Check sheet for the modelled part. Datum: model origin and axes. Units: mm. A direction names the side the tool comes from. Round coordinates to 2 decimals unless told otherwise and drop trailing zeros. Order: outer loops, then holes, each group sorted by start corner. A loop starts at its lowest first (then second) coordinate and runs counter-clockwise, first axis right, second up.
Autodesk Inventor part; units mm, degrees
ref_plane "YZ Plane" through (0, 0, 0) normal (1, 0, 0) x (0, 1, 0)
ref_plane "XZ Plane" through (0, 0, 0) normal (0, 1, 0) x (-1, 0, 0)
ref_plane "XY Plane" through (0, 0, 0) normal (0, 0, 1) x (1, 0, 0)
sketch "Skizze1" plane through (0, 0, 0) normal (0, 1, 0) x (-1, 0, 0)
  line L0 (39.8687, 22.5) -> (39.8687, 24)
  line L1 (39.8687, 24) -> (37.8687, 24)
  line L2 (37.8687, 24) -> (37.8687, 25)
  line L3 (37.8687, 25) -> (36.3687, 25)
  line L4 (36.3687, 22) -> (24.8687, 18.0718)
  line L5 (24.8687, 18.0718) -> (24.8687, 17.0718)
  line L6 (24.8687, 17.0718) -> (23.8687, 17.0718)
  line L7 (23.8687, 17.0718) -> (23.8687, 19)
  line L8 (23.8687, 19) -> (16.8687, 19)
  line L9 (16.8687, 19) -> (16.8687, 18)
  line L10 (16.8687, 18) -> (15.8687, 18)
  line L11 (15.8687, 18) -> (15.8687, 0)
  line L12 (39.8687, 22.5) -> (37.3687, 22.5)
  arc A0 (37.3687, 18.5) -> (37.3687, 22.5) centre (37.3687, 20.5) ccw
  line L13 (37.3687, 18.5) -> (30.1519, 6)
  arc A1 (32.1519, 0) -> (30.1519, 6) centre (22.1519, 0) ccw
  line L14 (0, -5) -> (0, 30) construction
  line L15 (-7.9737, 0) -> (47.8425, 0) construction
  line L16 (37.3687, 22.5) -> (37.3687, 18.5) construction
  line L17 (32.1519, 0) -> (15.8687, 0)
  line L18 (36.3687, 25) -> (36.3687, 22)
  point P0 (0, 0)
  dimension "d1" = 2
  dimension "d2" = 30
  dimension "d3" = 6
  dimension "d4" = 22.5
  dimension "d5" = 24
  dimension "d6" = 2
  dimension "d7" = 1
  dimension "d8" = 24
  dimension "d10" = 18
  dimension "d11" = 7
  dimension "d13" = 1
  dimension "d14" = 1
  dimension "d16" = 1
  dimension "d17" = 1.5
  dimension "d18" = 2
  dimension "d19" = 2.5
  dimension "d20" = 1
  dimension "d23" = 3
revolve "Umdrehung1" add sketch "Skizze1" angle 360 about axis through (0, 0, 0) along (-1, 0, 0)
properties part number "Loudspeaker"
1) Sectioned sample at C-C on x = -34.5. Record the cut outline in (y, z).
2) Scan lines: line 1 (X direction, y = 15, z = -17); line 2 (Y direction, x = -34, z = 1); line 3 (X direction, y = 23, z = -8). Record each from-to range of solid material in increasing order.
3) Set-up check for faces 1 (the face through (-20.32, 16.856, 8.767)), 2 (the face through (-38.855, -1.055, -23.977)), 3 (the face through (-15.869, 0, 0)), 4 (the face through (-37.108, -7.509, 23.846)), 5 (the face through (-25.588, -17.882, -3.971)): record each of +Z, -Z, +X, -X, +Y, -Y from which the full face is reachable in a straight line by a thin tool's end or side.
4) Gauge pin test, flat ends, axial feed: pin 1 (2 mm diameter, centred on x = -34, y = -16, fed in from +Z); pin 2 (4 mm diameter, centred on x = -30, y = 13.5, fed in from -Z); pin 3 (1 mm diameter, centred on x = -19.5, y = -7, fed in from +Z); pin 4 (12 mm diameter, centred on y = 17, z = 16, fed in from +X). Record the tip position at first contact, or that the pin passes through.
5) Draft check along X on faces 6 (the face through (-24.869, -16, 7)), 7 (the face through (-36.369, -22.1, 1.7)), 8 (the face through (-30.603, -6.621, -1.47)). Enter one of: pulls with the +X half, pulls with the -X half, needs draft (parallel to the pull), parting line crosses it, or undercut.
Values found:
1. outline: circle Ø42.72 at (0, 0); hole circle Ø27.06 at (0, 0)
2. line 1: x = -39.87 to -36.37
2. line 2: y = -21.17 to -12.63, 12.63 to 21.17
2. line 3: x = -37.87 to -36.37
3. face 1: +X
3. face 2: -X
3. face 3: +Z, -Z, +X, +Y, -Y
3. face 4: +X, -X
3. face 5: none
4. pin 1: stops at z = 15.08
4. pin 2: stops at z = -16.38
4. pin 3: stops at z = 17.85
4. pin 4: stops at x = -15.87
5. face 6: undercut
5. face 7: pulls with the +X half
5. face 8: pulls with the -X half
